from build123d import *

# Parameters (mm, degrees)
SKETCH1_W           = 117
SKETCH1_H           = 72
SKETCH1_W_2         = 111
SKETCH1_H_2         = 66
SKETCH1_W_3         = 110
SKETCH1_H_3         = 65
BOSS_EXTRUDE1_DEPTH = 3
SKETCH1_5_W         = 117
SKETCH1_5_H         = 72
SKETCH1_5_W_2       = 111
SKETCH1_5_H_2       = 66
BOSS_EXTRUDE2_DEPTH = 10
BOSS_EXTRUDE3_DEPTH = 3.85
SKETCH3_R           = 2
CUT_EXTRUDE1_DEPTH  = 4.78
FILLET1_R           = 2
SKETCH4_W           = 10
SKETCH4_H           = 8.13
CUT_EXTRUDE2_DEPTH  = 134.372598385
SKETCH5_W           = 10
SKETCH5_H           = 8.13
CUT_EXTRUDE3_DEPTH  = 134.203791237


with BuildPart() as part:
    # Sketch1 → Boss-Extrude1 (new body)
    with BuildSketch(Plane(origin=(0, 0, 0), x_dir=(1, 0, 0), z_dir=(0, 1, 0))):
        with Locations((55, 32.5)):
            Rectangle(SKETCH1_W, SKETCH1_H)
        with Locations((55, 32.5)):
            Rectangle(SKETCH1_W_2, SKETCH1_H_2, mode=Mode.SUBTRACT)
        with Locations((55, 32.5)):
            Rectangle(SKETCH1_W_2, SKETCH1_H_2)
        with Locations((55, 32.5)):
            Rectangle(SKETCH1_W_3, SKETCH1_H_3, mode=Mode.SUBTRACT)
        with Locations((55, 32.5)):
            Rectangle(SKETCH1_W_3, SKETCH1_H_3)
    extrude(amount=-BOSS_EXTRUDE1_DEPTH)

    # Sketch1_5 → Boss-Extrude2 (add)
    with BuildSketch(Plane(origin=(0, 0, 0), x_dir=(1, 0, 0), z_dir=(0, 1, 0))):
        with Locations((55, 32.5)):
            Rectangle(SKETCH1_5_W, SKETCH1_5_H)
        with Locations((55, 32.5)):
            Rectangle(SKETCH1_5_W_2, SKETCH1_5_H_2, mode=Mode.SUBTRACT)
    extrude(amount=BOSS_EXTRUDE2_DEPTH)

    # Sketch2 → Boss-Extrude3 (add)
    with BuildSketch(Plane(origin=(0, 0, 0), x_dir=(1, 0, 0), z_dir=(0, 1, 0))):
        with BuildLine():
            Line((110.5, 65.5), (100, 65.5))
            Line((100, 65.5), (100, 60))
            ThreePointArc((100, 60), (101.464466094, 56.464466094), (105, 55))
            Line((105, 55), (110.5, 55))
            Line((110.5, 55), (110.5, 65.5))
        make_face()
        with BuildLine():
            Line((-0.5, -0.5), (10, -0.5))
            Line((10, -0.5), (10, 5))
            ThreePointArc((10, 5), (8.535533906, 8.535533906), (5, 10))
            Line((5, 10), (-0.5, 10))
            Line((-0.5, 10), (-0.5, -0.5))
        make_face()
    extrude(amount=BOSS_EXTRUDE3_DEPTH)

    # Sketch3 → Cut-Extrude1 (cut)
    with BuildSketch(Plane(origin=(0, 3.85, 0), x_dir=(1, 0, 0), z_dir=(0, 1, 0))):
        with Locations(Location((105, 60, 0), (0, 0, 270))):
            Circle(SKETCH3_R)
        with Locations(Location((5, 5, 0), (0, 0, 270))):
            Circle(SKETCH3_R)
    extrude(amount=-CUT_EXTRUDE1_DEPTH, mode=Mode.SUBTRACT)

    # Fillet1
    fillet1_edges = [part.edges().sort_by_distance(p)[0] for p in [
        (-3.5, 3.5, -68.5),
        (113.5, 3.5, -68.5),
        (113.5, 3.5, 3.5),
        (-3.5, 3.5, 3.5),
    ]]
    fillet(fillet1_edges, radius=FILLET1_R)

    # Sketch4 → Cut-Extrude2 (cut, through all)
    with BuildSketch(Plane.ZY.offset(-110.5)):
        with Locations((-42.5, 5.935)):
            Rectangle(SKETCH4_W, SKETCH4_H)
    extrude(amount=-CUT_EXTRUDE2_DEPTH, mode=Mode.SUBTRACT)

    # Sketch5 → Cut-Extrude3 (cut, through all)
    with BuildSketch(Plane(origin=(0, 0, 0.5), x_dir=(-1, 0, 0), z_dir=(0, 0, -1))):
        with Locations((-78, 5.935)):
            Rectangle(SKETCH5_W, SKETCH5_H)
        with Locations((-48, 5.935)):
            Rectangle(SKETCH5_W, SKETCH5_H)
    extrude(amount=-CUT_EXTRUDE3_DEPTH, mode=Mode.SUBTRACT)


solid = part.part
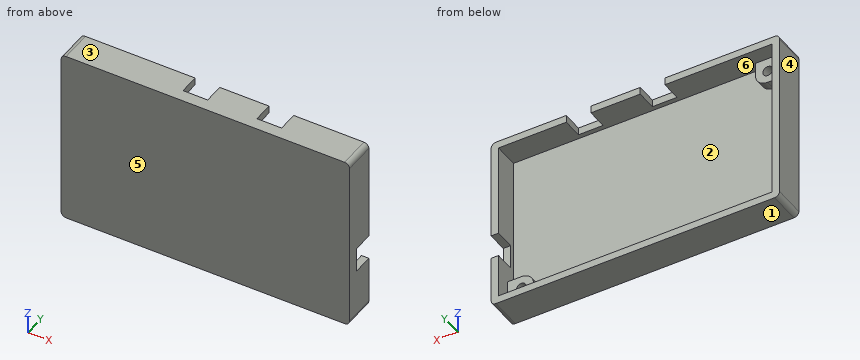
Read the model definition and answer for the solid it produces. Units are mm, in the model's axes. Face numbers are marked on the shaded views. A direction names the side the tool comes from. Coordinates: 2 decimals unless noted, no trailing zeros. Order: outer loops, then holes, each group sorted by start corner. A loop starts at its lowest first (then second) coordinate and runs counter-clockwise, first axis right, second up. Notation, with made-up numbers: M 75,6.5 L 99,6.5 A24 cw 99,22.5 Z; hole C 31,2 d5. An arc over 180 degrees is marked long. Put each result on its own line as item: value. Start each with the question number.
Item 1: The mould has two halves that part along Z. Classify the marked faces 1, 2, 3 and 4: +Z half, -Z half, draft (parallel to the pull), parting line (faces both ways), or undercut.
Item 2: Given pin 1 Ø3 at (x, z) = (51, -12.5) entering from +Y; pin 2 Ø2 at (x, z) = (104.5, -60) entering from +Y; pin 3 Ø2.5 at (y, z) = (4.5, 2.5) entering from +X; pin 4 Ø3.5 at (x, z) = (77.5, 2.5) entering from +Y, each flat-ended and moving along its own axis, determine where each tip first touches the part or whether it passes through.
Item 3: Consider probe 1 along X at (y, z) = (2.6, -60); probe 2 along X at (y, z) = (2.2, -5); probe 3 along X at (y, z) = (7.5, -28). Determine where each line is inside the solid, lowest interval first. Write a range as [from, to].
Item 4: Section B-B, the plane z = -13.5 is taken. Determine the outline of the cut face in (x, y).
Item 5: Section A-A, the plane y = 5 is taken. Determine the outline of the cut face in (x, z).
Item 6: For the marked faces 5 and 6, determine the directions among +Z, -Z, +X, -X, +Y, -Y from which every point of the face is accessible in a straight line to the end or side of a thin tool.
Item 7: Section C-C, the plane x = 11.5 is taken. Determine the outline of the cut face in (y, z), plus the area to 3 significant figures.
Computed:
1. face 1: -Z half
1. face 2: undercut
1. face 3: +Z half
1. face 4: draft
2. pin 1: stops at y = 0
2. pin 2: stops at y = -0.93
2. pin 3: stops at x = 113.5
2. pin 4: stops at y = 1.87
3. probe 1: x = [-3.5, -0.5], [100, 103], [107, 113.5]
3. probe 2: x = [-3.5, 3], [7, 10], [110.5, 113.5]
3. probe 3: x = [-3.5, -0.5], [110.5, 113.5]
4. outline: M -3.5,-3 L 113.5,-3 L 113.5,10 L 110.5,10 L 110.5,0 L -0.5,0 L -0.5,10 L -3.5,10 Z
5. outline: M -3.5,-66.5 A2 ccw -1.5,-68.5 L 111.5,-68.5 A2 ccw 113.5,-66.5 L 113.5,-47.5 L 110.5,-47.5 L 110.5,-65.5 L -0.5,-65.5 L -0.5,0.5 L 43,0.5 L 43,3.5 L -1.5,3.5 A2 ccw -3.5,1.5 Z; M 53,0.5 L 73,0.5 L 73,3.5 L 53,3.5 Z; M 83,0.5 L 110.5,0.5 L 110.5,-37.5 L 113.5,-37.5 L 113.5,1.5 A2 ccw 111.5,3.5 L 83,3.5 Z
6. face 5: +Z, -Z, +X, -X, -Y
6. face 6: +Y
7. outline: M -3,-68.5 L 10,-68.5 L 10,-65.5 L 0,-65.5 L 0,0.5 L 10,0.5 L 10,3.5 L -3,3.5 Z
7. area: 276 mm2
